from build123d import *

# Parameters (mm, degrees)
F0_W     = 10
F0_H     = 160
F0_W_2   = 160
F0_H_2   = 10
F0_R     = 8.5
F1_DEPTH = 2
F2_DEPTH = 20
F3_SIZE2 = 1.4558809371
F3_SIZE  = 4


with BuildPart() as f1:
    # F0 (on Front) → F1 (new body)
    with BuildSketch(Plane.XZ):
        with Locations((15, 100)):
            Rectangle(F0_W, F0_H)
        with Locations((-100, 15)):
            Rectangle(F0_W_2, F0_H_2)
        Polygon((-10, -20), (20, -20), (20, -10), (20, 20), (10, 20), (-20, 20), (-20, 10), (-20, -20), align=None)
        Circle(F0_R, mode=Mode.SUBTRACT)
        with Locations((100, -15)):
            Rectangle(F0_W_2, F0_H_2)
        with Locations((-15, -100)):
            Rectangle(F0_W, F0_H)
    extrude(amount=F1_DEPTH)

    # F0 (on Front) → F2 (join)
    with BuildSketch(Plane.XZ):
        Polygon((-10, -20), (20, -20), (20, -10), (20, 20), (10, 20), (-20, 20), (-20, 10), (-20, -20), align=None)
        Circle(F0_R, mode=Mode.SUBTRACT)
    extrude(amount=-F2_DEPTH)

    # F3
    f3_edges = [f1.edges().sort_by_distance(p)[0] for p in [
        (-85, -2, 20),
        (20, -2, 85),
        (85, -2, -20),
        (-20, -2, -85),
    ]]
    f3_side = f1.faces().sort_by_distance((15, -2, 174.908831))[0]
    chamfer(f3_edges, length=F3_SIZE, length2=F3_SIZE2, reference=f3_side)


solid = f1.part
Geometry check sheet. Reference: the model listing, model coordinates, mm. A direction names the side the tool comes from. Give positions to 0.01 mm unless a question says otherwise; leave off trailing zeros. Loops run counter-clockwise (first coordinate to the right, second up) from the corner with the lowest first, then second, coordinate; pieces in that order, holes last. Notation, with made-up numbers: M 1,-35.75 L 37,-35.75 A13 ccw 37,-22.75 Z; hole C 14.25,88.5 d2. An arc over 180 degrees is marked long. Write each question's results on one line, items separated by ' | '.
1) Release check for a two-part mould opening along X. For faces 1 (the face through (-15, 0, -99)), 2 (the face through (4.57, 9.154, 7.167)) record: +X half, -X half, draft (parallel to the pull), parting line (faces both ways), or undercut.
Answers follow:
face 1: draft | face 2: undercut
2) Gauge pin test, flat ends, axial feed: pin 1 (8 mm diameter, centred on x = -128.5, z = 15, fed in from +Y); pin 2 (13.5 mm diameter, centred on x = 0, z = 0, fed in from -Y); pin 3 (0.6 mm diameter, centred on x = -120.5, y = -1.5, fed in from -Z); pin 4 (2 mm diameter, centred on x = 94.5, y = -1.5, fed in from +Z). Record the tip position at first contact, or that the pin passes through.
Answers follow:
pin 1: y = 0 | pin 2: through | pin 3: z = 10 | pin 4: z = -10
3) Section check B-B, the plane x = 0. Record the boundary of the cut face in (y, z), plus the area to 3 significant figures.
Answers follow:
outline: M -2,-16 L -0.54,-20 L 20,-20 L 20,-8.5 L -2,-8.5 Z; M -2,8.5 L 20,8.5 L 20,20 L -0.54,20 L -2,16 Z | area: 500 mm2
4) Section check D-D, the plane z = 74. Record the boundary of the cut face in (x, y).
Answers follow:
outline: M 10,-2 L 16,-2 L 20,-0.54 L 20,0 L 10,0 Z
5) Section check A-A, the plane z = 0. Record the boundary of the cut face in (x, y), plus the area to 3 significant figures.
Answers follow:
outline: M -20,-0.54 L -16,-2 L -8.5,-2 L -8.5,20 L -20,20 Z; M 8.5,-2 L 16,-2 L 20,-0.54 L 20,20 L 8.5,20 Z | area: 500 mm2
6) Section check C-C, the plane y = 14.25. Record the boundary of the cut face in (x, z).
Answers follow:
outline: M -20,-20 L 20,-20 L 20,20 L -20,20 Z; hole C 0,0 d17
7) Tool access check on faces 3 (the face through (15, 0, 101)), 4 (the face through (99, 0, -15)), 5 (the face through (-14, -2, 1)), 6 (the face through (9, 20, 0)), 7 (the face through (-101, 0, 15)). Record the directions out of +Z, -Z, +X, -X, +Y, -Y that give a thin tool (end or side, any length) a straight path to the whole face; none if there is none.
Answers follow:
face 3: +Z, +X, -X, +Y | face 4: +Z, -Z, +X, +Y | face 5: +Z, -Z, +X, -X, -Y | face 6: +Z, -Z, +X, -X, +Y | face 7: +Z, -Z, -X, +Y
8) Thickness scan on line 1 (Z direction, x = 0, y = 4.5); line 2 (X direction, y = 6.5, z = -10); line 3 (Z direction, x = 2, y = 7.25). Record the ranges inside material, lowest first.
Answers follow:
line 1: -20 to -8.5, 8.5 to 20 | line 2: -20 to 20 | line 3: -20 to -8.26, 8.26 to 20
